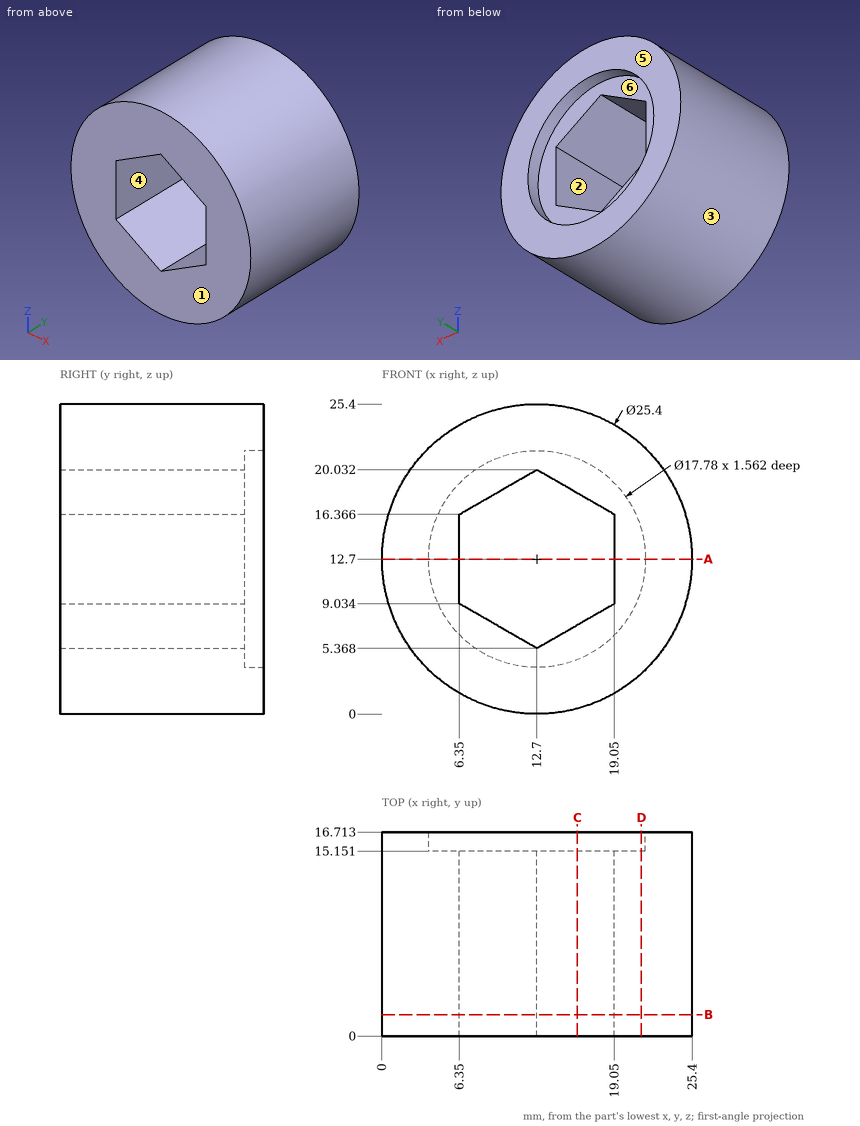
Geometry: see drawing. Coordinates: mm, zero at the bounding-box minimum. A direction names the side the tool comes from. Give positions to 0.01 mm unless a question says otherwise; leave off trailing zeros. Loops run counter-clockwise (first coordinate to the right, second up) from the corner with the lowest first, then second, coordinate; pieces in that order, holes last. Notation, with made-up numbers: (12, -24.5) -> (56, -24.5) arc R30 cw to (56, -0.5) -> close; hole circle Ø1 at (70, 85.5). An arc over 180 degrees is marked (long way). Use CSV: the item, a comma, the result in double quotes.
(1) Cut plane A-A (z = 12.7). Output: boundary loops of the cut face in (x, y).
From the geometry:
outline,"(0, 0) -> (6.35, 0) -> (6.35, 15.15) -> (3.81, 15.15) -> (3.81, 16.71) -> (0, 16.71) -> close; (19.05, 0) -> (25.4, 0) -> (25.4, 16.71) -> (21.59, 16.71) -> (21.59, 15.15) -> (19.05, 15.15) -> close"
(2) Access query for the marked faces 4, 5 and 6. Directions: +Z, -Z, +X, -X, +Y, -Y. A direction counts if a zero-diameter tool reaches every point of the face in a straight line with its end or side. Return the directions, or none.
From the geometry:
face 4,"+Y, -Y"
face 5,"+Z, -Z, +X, -X, +Y"
face 6,"+Y"
(3) Cut plane D-D (x = 21.25). Output: boundary loops of the cut face in (y, z) (1 decimal).
From the geometry:
outline,"(0, 3.3) -> (16.7, 3.3) -> (16.7, 10.3) -> (15.2, 10.3) -> (15.2, 15.1) -> (16.7, 15.1) -> (16.7, 22.1) -> (0, 22.1) -> close"
(4) First-contact query: P1, Ø1.5, axis at x = 21, z = 20.5, coming from the -Y side; P2, Ø1.5, axis at x = 18, y = 7.5, coming from the +Z side; P3, Ø3, axis at y = 5.5, z = 21, coming from the -X side; P4, Ø4, axis at x = 6, y = 7.5, coming from the -Z side. Flat tips, straight axial feed; report the tip coordinate or a pass-through.
From the geometry:
P1,"y = 0"
P2,"z = 24.56"
P3,"x = 1.97"
P4,"z = 0.9"
(5) Cut plane B-B (y = 1.75). Output: boundary loops of the cut face in (x, z).
From the geometry:
outline,"circle Ø25.4 at (12.7, 12.7); hole (6.35, 9.03) -> (12.7, 5.37) -> (19.05, 9.03) -> (19.05, 16.37) -> (12.7, 20.03) -> (6.35, 16.37) -> close"
(6) Ray query, line 1 along X through (y, z) = (16, 12.7); line 2 along X through (y, z) = (6.25, 8.5) (1 decimal). Return the intervals inside material, ascending. Write a range as [from, to].
From the geometry:
line 1,"[0, 3.81], [21.59, 25.4]"
line 2,"[0.7, 7.3], [18.1, 24.7]"
(7) Pull-direction query (X, two-part tool) for the marked faces 1, 2 and 3; classes: released by +X, released by -X, zero draft, split by the parting line, or undercut.
From the geometry:
face 1,"zero draft"
face 2,"undercut"
face 3,"split by the parting line"
(8) Cut plane C-C (x = 16). Output: boundary loops of the cut face in (y, z) (1 decimal), plus the area to 3 significant figures.
From the geometry:
outline,"(0, 0.4) -> (16.7, 0.4) -> (16.7, 4.4) -> (15.2, 4.4) -> (15.2, 7.3) -> (0, 7.3) -> close; (0, 18.1) -> (15.2, 18.1) -> (15.2, 21) -> (16.7, 21) -> (16.7, 25) -> (0, 25) -> close"
area,"220 mm^2"
